Read the model definition and answer for the solid it produces. Units are mm, in the model's axes. A direction names the side the tool comes from. Give positions to 0.01 mm unless a question says otherwise; leave off trailing zeros. Write each question's results on one line, items separated by ' | '. Start each with the question number.
Q1. Determine the mould class of faces 4 (the flat face through (20, 34, 5)), 5 (the conical face through (2.183, 61.003, 5.16)), 6 (the flat face through (10, 0, 5)) for opening direction X: +X half, -X half, draft (parallel to the pull), parting line (faces both ways), or undercut.
Q2. Find the intervals of material crossed by line 1 (X direction, y = 2.75, z = 5); line 2 (X direction, y = 67.75, z = 5); line 3 (Z direction, x = 15, y = 3.75), in increasing order. Write a range as from..to.
Q3. Given pin 1 (1.5 mm diameter, centred on x = 15, z = 5, fed in from -Y); pin 2 (1 mm diameter, centred on x = 2.5, y = 20.5, fed in from -Z), each flat-ended and moving along its own axis, determine where each tip first touches the part or whether it passes through.
Q4. For faces 1 (the flat face through (0, 35, 5)), 2 (the cylindrical face through (18.726, 65.444, 4.783)), 3 (the cylindrical face through (13.76, 4.06, 5.16)), determine the directions among +Z, -Z, +X, -X, +Y, -Y from which every point of the face is accessible in a straight line to the end or side of a thin tool.
Autodesk Inventor part; units mm, degrees
ref_plane "YZ Plane" through (0, 0, 0) normal (1, 0, 0) x (0, 1, 0)
ref_plane "XZ Plane" through (0, 0, 0) normal (0, 1, 0) x (-1, 0, 0)
ref_plane "XY Plane" through (0, 0, 0) normal (0, 0, 1) x (1, 0, 0)
sketch "Skizze1" plane through (0, 0, 0) normal (0, 0, 1) x (1, 0, 0)
  line L0 (0, 0) -> (20, 0)
  line L1 (20, 0) -> (20, 69.5)
  line L2 (20, 69.5) -> (0, 69.5)
  line L3 (0, 69.5) -> (0, 0)
  dimension "d0" = 20
  dimension "d1" = 69.5
extrude "Extrusion1" add sketch "Skizze1" along normal blind 10
sketch "Skizze2" plane through (0, 69.5, 0) normal (0, 1, 0) x (1, 0, 0)
  line L0 (20, 0) -> (20, -10)
  line L1 (20, -10) -> (20, -5)
  line L2 (20, -5) -> (17.75, -5)
  line L3 (17.75, -5) -> (2.25, -5)
  point P0 (0, 0)
  dimension "d4" = 2.25
  dimension "d5" = 15.5
hole "Bohrung1" at (2.25, 69.5, 5) at (17.75, 69.5, 5) direction (0, -1, 0) diameter 2 depth 8 tip angle 118
sketch "Skizze3" plane through (0, 0, 0) normal (0, -1, 0) x (1, 0, 0)
  line L0 (20, 10) -> (0, 10)
  line L1 (0, 10) -> (0, 5)
  line L2 (0, 0) -> (0, 10)
  line L3 (0, 5) -> (5, 5)
  line L4 (5, 5) -> (15, 5)
  dimension "d13" = 5
  dimension "d14" = 10
hole "Bohrung2" at (5, 0, 5) at (15, 0, 5) direction (0, 1, 0) diameter 2.5 depth 8 tip angle 118
properties part number "Sensor_Halterung_Drehplatte" material "Holz (Eiche)"
Check sheet entries:
1) face 4: +X half | face 5: undercut | face 6: draft
2) line 1: x = 0..3.75, 6.25..13.75, 16.25..20 | line 2: x = 0..1.25, 3.25..16.75, 18.75..20 | line 3: z = 0..3.75, 6.25..10
3) pin 1: stops at y = 8.3 | pin 2: stops at z = 0
4) face 1: +Z, -Z, -X, +Y, -Y | face 2: +Y | face 3: -Y
